```python
from build123d import *

# Parameters (mm, degrees)
SKETCH1_W           = 90
SKETCH1_H           = 75
BOSS_EXTRUDE1_DEPTH = 5
SKETCH2_W           = 90
SKETCH2_H           = 5
BOSS_EXTRUDE2_DEPTH = 15
SKETCH3_W           = 5
SKETCH3_H           = 15
BOSS_EXTRUDE3_DEPTH = 70
CUT_EXTRUDE1_REACH  = 92
SKETCH5_R           = 1.6
CUT_EXTRUDE3_REACH  = 77
SKETCH7_R           = 1.6
SKETCH8_W           = 50.1
SKETCH8_H           = 57.079275331
BOSS_EXTRUDE6_DEPTH = 3
CUT_EXTRUDE4_REACH  = 10
SKETCH9_R           = 1.6
CUT_EXTRUDE5_START  = -2.5
CUT_EXTRUDE5_DEPTH  = 2.5
BOSS_EXTRUDE7_DEPTH = 7.5
SKETCH12_W          = 5
SKETCH12_H          = 10
BOSS_EXTRUDE8_DEPTH = 17.5
CUT_EXTRUDE6_REACH  = 92
SKETCH13_R          = 1.6


with BuildPart() as part:
    # Sketch1 → Boss-Extrude1 (new body)
    with BuildSketch(Plane(origin=(0, 0, 0), x_dir=(1, 0, 0), z_dir=(0, 1, 0))):
        Rectangle(SKETCH1_W, SKETCH1_H)
    extrude(amount=BOSS_EXTRUDE1_DEPTH)

    # Sketch2 → Boss-Extrude2 (add)
    with BuildSketch(Plane(origin=(0, 5, 0), x_dir=(1, 0, 0), z_dir=(0, 1, 0))):
        with Locations((0, -35)):
            Rectangle(SKETCH2_W, SKETCH2_H)
    extrude(amount=BOSS_EXTRUDE2_DEPTH)

    # Sketch3 → Boss-Extrude3 (add)
    with BuildSketch(Plane(origin=(0, 0, 32.5), x_dir=(-1, 0, 0), z_dir=(0, 0, -1))):
        with Locations((-42.5, 12.5)):
            Rectangle(SKETCH3_W, SKETCH3_H)
    extrude(amount=BOSS_EXTRUDE3_DEPTH)

    # Sketch5 → Cut-Extrude1 (cut, up to next)
    with BuildSketch(Plane(origin=(45, 0, 0), x_dir=(0, 0, -1), z_dir=(1, 0, 0)), mode=Mode.PRIVATE) as cut_extrude1_sk1:
        with Locations((-2.5, 13.75)):
            Circle(SKETCH5_R)
    cut_extrude1_tool1 = extrude(cut_extrude1_sk1.sketch, amount=-CUT_EXTRUDE1_REACH, mode=Mode.PRIVATE) & part.part
    add(cut_extrude1_tool1.solids().sort_by_distance((45, 13.75, 2.5))[0], mode=Mode.SUBTRACT)
    # Sketch5 → Cut-Extrude1 (cut, up to next)
    with BuildSketch(Plane(origin=(45, 0, 0), x_dir=(0, 0, -1), z_dir=(1, 0, 0)), mode=Mode.PRIVATE) as cut_extrude1_sk2:
        with Locations((32.5, 13.75)):
            Circle(SKETCH5_R)
    cut_extrude1_tool2 = extrude(cut_extrude1_sk2.sketch, amount=-CUT_EXTRUDE1_REACH, mode=Mode.PRIVATE) & part.part
    add(cut_extrude1_tool2.solids().sort_by_distance((45, 13.75, -32.5))[0], mode=Mode.SUBTRACT)

    # Sketch7 → Cut-Extrude3 (cut, up to next)
    with BuildSketch(Plane.XY.offset(37.5), mode=Mode.PRIVATE) as cut_extrude3_sk1:
        with Locations((-15, 13.75)):
            Circle(SKETCH7_R)
    cut_extrude3_tool1 = extrude(cut_extrude3_sk1.sketch, amount=-CUT_EXTRUDE3_REACH, mode=Mode.PRIVATE) & part.part
    add(cut_extrude3_tool1.solids().sort_by_distance((-15, 13.75, 37.5))[0], mode=Mode.SUBTRACT)
    # Sketch7 → Cut-Extrude3 (cut, up to next)
    with BuildSketch(Plane.XY.offset(37.5), mode=Mode.PRIVATE) as cut_extrude3_sk2:
        with Locations((15, 13.75)):
            Circle(SKETCH7_R)
    cut_extrude3_tool2 = extrude(cut_extrude3_sk2.sketch, amount=-CUT_EXTRUDE3_REACH, mode=Mode.PRIVATE) & part.part
    add(cut_extrude3_tool2.solids().sort_by_distance((15, 13.75, 37.5))[0], mode=Mode.SUBTRACT)

    # Sketch8 → Boss-Extrude6 (add)
    with BuildSketch(Plane(origin=(0, 5, 0), x_dir=(1, 0, 0), z_dir=(0, 1, 0))):
        with Locations((-9.469239884, 8.960362334)):
            Rectangle(SKETCH8_W, SKETCH8_H)
    extrude(amount=BOSS_EXTRUDE6_DEPTH)

    # Sketch9 → Cut-Extrude4 (cut, up to next)
    with BuildSketch(Plane(origin=(0, 8, 0), x_dir=(1, 0, 0), z_dir=(0, 1, 0)), mode=Mode.PRIVATE) as cut_extrude4_sk1:
        with Locations((-24.419239884, 12.920724669)):
            Circle(SKETCH9_R)
    cut_extrude4_tool1 = extrude(cut_extrude4_sk1.sketch, amount=-CUT_EXTRUDE4_REACH, mode=Mode.PRIVATE) & part.part
    add(cut_extrude4_tool1.solids().sort_by_distance((-24.41924, 8, -12.920725))[0], mode=Mode.SUBTRACT)
    # Sketch9 → Cut-Extrude4 (cut, up to next)
    with BuildSketch(Plane(origin=(0, 8, 0), x_dir=(1, 0, 0), z_dir=(0, 1, 0)), mode=Mode.PRIVATE) as cut_extrude4_sk2:
        with Locations((5.480760116, 12.920724669)):
            Circle(SKETCH9_R)
    cut_extrude4_tool2 = extrude(cut_extrude4_sk2.sketch, amount=-CUT_EXTRUDE4_REACH, mode=Mode.PRIVATE) & part.part
    add(cut_extrude4_tool2.solids().sort_by_distance((5.48076, 8, -12.920725))[0], mode=Mode.SUBTRACT)
    # Sketch9 → Cut-Extrude4 (cut, up to next)
    with BuildSketch(Plane(origin=(0, 8, 0), x_dir=(1, 0, 0), z_dir=(0, 1, 0)), mode=Mode.PRIVATE) as cut_extrude4_sk3:
        with Locations((5.480760116, -2.079275331)):
            Circle(SKETCH9_R)
    cut_extrude4_tool3 = extrude(cut_extrude4_sk3.sketch, amount=-CUT_EXTRUDE4_REACH, mode=Mode.PRIVATE) & part.part
    add(cut_extrude4_tool3.solids().sort_by_distance((5.48076, 8, 2.079275))[0], mode=Mode.SUBTRACT)
    # Sketch9 → Cut-Extrude4 (cut, up to next)
    with BuildSketch(Plane(origin=(0, 8, 0), x_dir=(1, 0, 0), z_dir=(0, 1, 0)), mode=Mode.PRIVATE) as cut_extrude4_sk4:
        with Locations((-24.519239884, -2.079275331)):
            Circle(SKETCH9_R)
    cut_extrude4_tool4 = extrude(cut_extrude4_sk4.sketch, amount=-CUT_EXTRUDE4_REACH, mode=Mode.PRIVATE) & part.part
    add(cut_extrude4_tool4.solids().sort_by_distance((-24.51924, 8, 2.079275))[0], mode=Mode.SUBTRACT)

    # Sketch10 → Cut-Extrude5 (cut)
    with BuildSketch(Plane(origin=(0, 8, 0), x_dir=(1, 0, 0), z_dir=(0, 1, 0)).offset(CUT_EXTRUDE5_START)):
        Polygon((-21.091380421, -2.304248294), (-22.61047785, 0.776851563), (-26.038337313, 1.001824527), (-27.947099347, -1.854302367), (-26.428001917, -4.935402224), (-23.000142454, -5.160375188), align=None)
        Polygon((8.908619579, -2.304248294), (7.38952215, 0.776851563), (3.961662687, 1.001824527), (2.052900653, -1.854302367), (3.571998083, -4.935402224), (6.999857546, -5.160375188), align=None)
        Polygon((8.908619579, 12.695751706), (7.38952215, 15.776851563), (3.961662687, 16.001824527), (2.052900653, 13.145697633), (3.571998083, 10.064597776), (6.999857546, 9.839624812), align=None)
        Polygon((-20.991380369, 12.695752494), (-22.510478507, 15.776852002), (-25.938338022, 16.001824178), (-27.847099399, 13.145696845), (-26.328001261, 10.064597337), (-22.900141746, 9.839625161), align=None)
    extrude(amount=-CUT_EXTRUDE5_DEPTH, mode=Mode.SUBTRACT)

    # Sketch11 → Boss-Extrude7 (add)
    with BuildSketch(Plane(origin=(0, 0, -37.5), x_dir=(-1, 0, 0), z_dir=(0, 0, -1))):
        Polygon((-45, 20), (-45, 0), (45, 0), (45, 5), (34.519239884, 5), (34.519239884, 8), (-15.580760116, 8), (-15.580760116, 5), (-40, 5), (-40, 20), align=None)
    extrude(amount=BOSS_EXTRUDE7_DEPTH)

    # Sketch12 → Boss-Extrude8 (add)
    with BuildSketch(Plane(origin=(0, 5, 0), x_dir=(1, 0, 0), z_dir=(0, 1, 0))):
        with Locations((-42.5, 40)):
            Rectangle(SKETCH12_W, SKETCH12_H)
    extrude(amount=BOSS_EXTRUDE8_DEPTH)

    # Sketch13 → Cut-Extrude6 (cut, up to next)
    with BuildSketch(Plane.ZY.offset(45), mode=Mode.PRIVATE) as cut_extrude6_sk1:
        with Locations((-40, 15)):
            Circle(SKETCH13_R)
    cut_extrude6_tool1 = extrude(cut_extrude6_sk1.sketch, amount=-CUT_EXTRUDE6_REACH, mode=Mode.PRIVATE) & part.part
    add(cut_extrude6_tool1.solids().sort_by_distance((-45, 15, -40))[0], mode=Mode.SUBTRACT)


solid = part.part
```
The model under review builds one solid part; all positions refer to its coordinate system, in mm. A direction names the side the tool comes from. Give positions to 0.01 mm unless a question says otherwise; leave off trailing zeros. Loops run counter-clockwise (first coordinate to the right, second up) from the corner with the lowest first, then second, coordinate; pieces in that order, holes last. Notation, with made-up numbers: (-8.75, -23.5) - (-0.75, -23.5) arc R26 ccw to (-0.75, 3.5) - close; hole circle Ø11 at (17.25, -29). An arc over 180 degrees is marked (long way). Answer as a JSON object with one key per item and string values.
Q1. Add section B-B on x = -15. State the section outline as (y, z) points.
Worked out:
{"outline": "(0, -45) - (8, -45) - (8, 19.58) - (5, 19.58) - (5, 32.5) - (12.15, 32.5) - (12.15, 37.5) - (0, 37.5) - close; (15.35, 32.5) - (20, 32.5) - (20, 37.5) - (15.35, 37.5) - close"}
Q2. To check wall thickness, follow line 1 along X through (y, z) = (7, -35.5); line 2 along Z through (x, y) = (5.5, 1.75); line 3 along X through (y, z) = (6.5, -33). State the ranges of each line that lie inside material, in increasing order.
Worked out:
{"line 1": "x = -45 to -40, -34.52 to 15.58, 40 to 45", "line 2": "z = -45 to -14.52, -11.32 to 0.48, 3.68 to 37.5", "line 3": "x = -34.52 to 15.58, 40 to 45"}
Q3. Mouldability with a two-part tool opening along Z and no side actions: class faces 4 (the flat face through (-11, 6, -45)), 5 (the flat face through (1, 0, -3)), 6 (the cylindrical face through (-25.69, 6.77, -11.95)) as +Z half, -Z half, draft (parallel to the pull), parting line (faces both ways), or undercut.
Worked out:
{"face 4": "-Z half", "face 5": "draft", "face 6": "undercut"}
Q4. Add section D-D on x = -37. State the section outline as (y, z) points.
Worked out:
{"outline": "(0, -45) - (5, -45) - (5, 32.5) - (20, 32.5) - (20, 37.5) - (0, 37.5) - close"}
Q5. Add section A-A on z = -40. State the section outline as (x, y) points, plus the area to 3 significant figures.
Worked out:
{"outline": "(-45, 0) - (45, 0) - (45, 20) - (40, 20) - (40, 5) - (15.58, 5) - (15.58, 8) - (-34.52, 8) - (-34.52, 5) - (-40, 5) - (-40, 13.4) - (-45, 13.4) - close; (-45, 16.6) - (-40, 16.6) - (-40, 22.5) - (-45, 22.5) - close", "area": "747 mm^2"}
Q6. For faces 1 (the flat face through (45, 10, -3)), 2 (the flat face through (2.8, 4.27, 3.37)), 3 (the flat face through (40, 12, -6)), list the 3-axis set-ups (+Z, -Z, +X, -X, +Y, -Y) from which the entire face can be reached by the end or side of a thin tool; tool diameter is ignored.
Worked out:
{"face 1": "+Z, -Z, +X, +Y, -Y", "face 2": "none", "face 3": "-Z, +Y"}
Q7. Add section C-C on z = 12. State the section outline as (x, y) points, plus the area to 3 significant figures.
Worked out:
{"outline": "(-45, 0) - (45, 0) - (45, 20) - (40, 20) - (40, 5) - (15.58, 5) - (15.58, 8) - (-34.52, 8) - (-34.52, 5) - (-45, 5) - close", "area": "675 mm^2"}
Q8. Insertion check: pin 1 (1 mm diameter, centred on x = -31, z = -32.5, fed in from +Y); pin 2 (2.5 mm diameter, centred on x = 5.48, z = -12.92, fed in from -Y); pin 3 (1 mm diameter, centred on x = -12, y = 19, fed in from -Z); pin 4 (7.5 mm diameter, centred on y = 10, z = -3, fed in from -X). Each pin has a flat end and moves straight along its axis. Give the tip position at first contact, or say it passes through.
Worked out:
{"pin 1": "stops at y = 8", "pin 2": "passes through", "pin 3": "stops at z = 32.5", "pin 4": "stops at x = -34.52"}
